Read the model definition and answer for the solid it produces. Units are mm, in the model's axes. Face numbers are marked on the shaded views. A direction names the side the tool comes from. Give positions to 0.01 mm unless a question says otherwise; leave off trailing zeros. Write each loop counter-clockwise with the first axis right and the second up, starting at its lowest first coordinate (ties: lowest second). Pieces come first, ordered by that corner, then holes. Notation, with made-up numbers: (-37.75, 61) -> (1.25, 61) arc R11 ccw to (1.25, 79) -> close; hole circle Ø7 at (73.5, 49.25). An arc over 180 degrees is marked (long way). Write item = value, one per line.
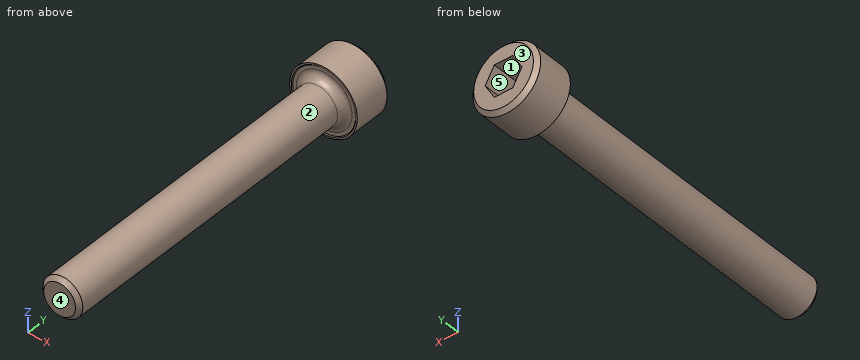
from build123d import *
from build123d.topology import SkipClean

# Parameters (mm, degrees)
CHAMFER1_SIZE      = 0.5
FILLET2_R          = 1
CUT_EXTRUDE1_DEPTH = 4


with BuildPart() as part:
    # Sketch1 → Revolve1 (revolve)
    with BuildSketch(Plane.XY, mode=Mode.PRIVATE) as revolve1_sk:
        Polygon((0, 0), (4.25, 0), (4.25, -5), (2.5, -5), (2.5, -45), (0, -45), align=None)
    revolve(revolve1_sk.sketch.rotate(Axis((0, -45, 0), (0, 1, 0)), 90), axis=Axis((0, -45, 0), (0, 1, 0)))

    # Chamfer1
    chamfer1_edges = [part.edges().sort_by_distance(p)[0] for p in [
        (0, -45, 2.5),
        (0, 0, 4.25),
    ]]
    chamfer(chamfer1_edges, length=CHAMFER1_SIZE)

    # Sketch2 → Cut-Revolve1 (revolve, cut)
    with SkipClean():  # the faces are left unmerged after this step: merging them gives an invalid solid
        with BuildSketch(Plane.XY, mode=Mode.PRIVATE) as cut_revolve1_sk:
            Polygon((3.95, -4.9), (2.5, -4.9), (2.5, -5.679573885), (4.05, -5.679573885), (4.05, -5), align=None)
        revolve(cut_revolve1_sk.sketch.rotate(Axis((0, 0, 0), (0, -1, 0)), 90), axis=Axis((0, 0, 0), (0, -1, 0)), mode=Mode.SUBTRACT)

    # Fillet2
    fillet2_edges = [part.edges().sort_by_distance(p)[0] for p in [
        (0, -4.9, -2.5),
    ]]
    fillet(fillet2_edges, radius=FILLET2_R)

    # Sketch3 → Cut-Extrude1 (cut)
    with BuildSketch(Plane(origin=(0, 0, 0), x_dir=(1, 0, 0), z_dir=(0, 1, 0))):
        Polygon((-1.154700538, 2), (-2.309401077, 0), (-1.154700538, -2), (1.154700538, -2), (2.309401077, 0), (1.154700538, 2), align=None)
    extrude(amount=-CUT_EXTRUDE1_DEPTH, mode=Mode.SUBTRACT)


solid = part.part
(1) The part is cut by section A-A on y = -36.5. Determine the outline of the cut face in (x, z), plus the area to 3 significant figures.
Checks:
outline = circle Ø5 at (0, 0)
area = 19.6 mm²
(2) For a pull along X with two mould halves and no side action, classify the marked faces 1, 2 and 3 as released by +X, released by -X, zero draft, split by the parting line, or undercut.
Checks:
face_1 = undercut
face_2 = split by the parting line
face_3 = zero draft
(3) Consider L1, parallel to Y at x = 0, z = 1.5; L2, parallel to X at y = -35.5, z = -1.5; L3, parallel to Z at x = -0.75, y = -1.5. Determine where each line is inside the solid, lowest interval first.
Checks:
L1 = -45 to -4
L2 = -2 to 2
L3 = -4.18 to -2, 2 to 4.18
(4) A tool of negligible diameter and unlimited length cuts with its end or side. For the marked faces 4 and 5, from which of +Z, -Z, +X, -X, +Y, -Y can it reach the whole face along a straight path? Write none if from no direction.
Checks:
face_4 = +Z, -Z, +X, -X, -Y
face_5 = +Y
(5) Given P1, Ø3, axis at y = -24, z = 2.5, coming from the +X side; P2, Ø2, axis at x = -0.5, y = -39.5, coming from the -Z side; P3, Ø0.7, axis at x = -0.5, y = -1, coming from the -Z side, each flat-ended and moving along its own axis, determine where each tip first touches the part or whether it passes through.
Checks:
P1 = 2.29
P2 = -2.5
P3 = -4.25
